Part model, mm, in its own coordinate system. Round coordinates to 2 decimals unless told otherwise and drop trailing zeros. Loops run counter-clockwise (first coordinate to the right, second up) from the corner with the lowest first, then second, coordinate; pieces in that order, holes last. Notation, with made-up numbers: (-36.5, 5) -> (-31.5, 5) arc R9 cw to (-31.5, 20) -> close; hole circle Ø5 at (22, -29.5). An arc over 180 degrees is marked (long way). Answer as CSV lines item,"result".
from build123d import *

# Parameters (mm, degrees)
SKETCH1_W           = 62.5
SKETCH1_H           = 10
BOSS_EXTRUDE1_DEPTH = 6
SKETCH2_R           = 1.65
CUT_EXTRUDE1_DEPTH  = 64.578691399
FILLET1_R           = 3


with BuildPart() as part:
    # Sketch1 → Boss-Extrude1 (new body)
    with BuildSketch(Plane.XY):
        with Locations((31.25, -5)):
            Rectangle(SKETCH1_W, SKETCH1_H)
    extrude(amount=BOSS_EXTRUDE1_DEPTH)

    # Sketch2 → Cut-Extrude1 (cut, through all)
    with BuildSketch(Plane.XY.offset(6)):
        with Locations((56.5, -5)):
            Circle(SKETCH2_R)
        with Locations((6, -5)):
            Circle(SKETCH2_R)
    extrude(amount=-CUT_EXTRUDE1_DEPTH, mode=Mode.SUBTRACT)

    # Fillet1
    fillet1_edges = [part.edges().sort_by_distance(p)[0] for p in [
        (0, 0, 3),
        (62.5, 0, 3),
        (62.5, -10, 3),
        (0, -10, 3),
    ]]
    fillet(fillet1_edges, radius=FILLET1_R)


solid = part.part
Q1. Saw through at A-A, the plane x = 56.5. Write the cut outline in (y, z).
Geometry results:
outline,"(-10, 0) -> (-6.65, 0) -> (-6.65, 6) -> (-10, 6) -> close; (-3.35, 0) -> (0, 0) -> (0, 6) -> (-3.35, 6) -> close"
Q2. Drop flat-ended pins along their axis: P1, Ø2, axis at y = -1.5, z = 4.5, coming from the +X side; P2, Ø2.5, axis at x = 56.5, y = -5, coming from the -Z side; P3, Ø1, axis at y = -2, z = 4.5, coming from the -X side. Give the stop position or say it passes through.
Geometry results:
P1,"x = 62.46"
P2,"through"
P3,"x = 0.04"
Q3. Two-plate mould, pull along X, no slides. Class faces 1 (the face through (0.86, -0.9, 3.04)), 2 (the face through (4.35, -4.93, 3.04)), 3 (the face through (31, -10, 3)): pulls with the +X half, pulls with the -X half, needs draft (parallel to the pull), parting line crosses it, or undercut.
Geometry results:
face 1,"pulls with the -X half"
face 2,"undercut"
face 3,"needs draft"
Q4. Saw through at C-C, the plane z = 1.8. Write the cut outline in (x, y).
Geometry results:
outline,"(0, -7) arc R3 ccw to (3, -10) -> (59.5, -10) arc R3 ccw to (62.5, -7) -> (62.5, -3) arc R3 ccw to (59.5, 0) -> (3, 0) arc R3 ccw to (0, -3) -> close; hole circle Ø3.3 at (6, -5); hole circle Ø3.3 at (56.5, -5)"
Q5. Drill centre lines: line 1 along Y through (x, z) = (6, 3.45); line 2 along X through (y, z) = (-3.5, 2.15); line 3 along X through (y, z) = (-5.5, 4.1). Where is each one in solid material? Low to high.
Geometry results:
line 1,"-10 to -6.65, -3.35 to 0"
line 2,"0 to 5.31, 6.69 to 55.81, 57.19 to 62.5"
line 3,"0 to 4.43, 7.57 to 54.93, 58.07 to 62.5"
Q6. Saw through at B-B, the plane y = -5. Write the cut outline in (x, z).
Geometry results:
outline,"(0, 0) -> (4.35, 0) -> (4.35, 6) -> (0, 6) -> close; (7.65, 0) -> (54.85, 0) -> (54.85, 6) -> (7.65, 6) -> close; (58.15, 0) -> (62.5, 0) -> (62.5, 6) -> (58.15, 6) -> close"
